Here's how the part is built. I have some questions about the finished solid (model axes, mm). Coordinates: 2 decimals unless noted, no trailing zeros. Order: outer loops, then holes, each group sorted by start corner. A loop starts at its lowest first (then second) coordinate and runs counter-clockwise, first axis right, second up. Notation, with made-up numbers: (83, -12.5) - (100, -12.5) arc R20 cw to (100, 19.5) - close; hole circle Ø10 at (18, 21). An arc over 180 degrees is marked (long way). Answer in a Markdown table with one row per item. Add a question column.
Item 1: I want a section at A-A (x = 31). Please give me the cut outline in (y, z).
Item 2: If I drill on line 1 along Y through (x, z) = (0, 0.7); line 2 along Y through (x, z) = (100, -0.65); line 3 along X through (y, z) = (-3.25, -1.2), over which ranges is the centre line in solid material (lowest first)? Write a range as from..to.
Item 3: I want a section at C-C (x = 93). Please give me the cut outline in (y, z), plus the area to 3 significant figures.
Item 4: Will this pin go through, and if not, where does the flat tip stop? pin 1 Ø1 at (y, z) = (9.5, -1) entering from -X.
Item 5: I want a section at D-D (y = -12.5). Please give me the cut outline in (x, z).
Item 6: I want a section at B-B (z = -0.85). Count the separate pieces of the cut face and the enclosed holes in it, plus the area to 3 significant figures.
```python
from build123d import *

# Parameters (mm, degrees)
BOSS_EXTRU_1_DEPTH      = 1.5
BOSS_EXTRU_1_DEPTH_BACK = 1.5
ESQUISSE1_R             = 0.8
ESQUISSE1_R_2           = 2.2
ESQUISSE1_R_3           = 4


with BuildPart() as part:
    # Esquisse1 → Boss.-Extru.1 (new, two sides: drawn at the far end of the back side and taken through both)
    with BuildSketch(Plane.XY.offset(-BOSS_EXTRU_1_DEPTH_BACK)):
        with BuildLine():
            Line((0, -15), (100, -10))
            ThreePointArc((100, -10), (110, 0), (100, 10))
            Line((100, 10), (0, 15))
            ThreePointArc((0, 15), (-15, 0), (0, -15))
        make_face()
        with Locations((5.656854249, 5.656854249)):
            Circle(ESQUISSE1_R, mode=Mode.SUBTRACT)
        with Locations((8, 0)):
            Circle(ESQUISSE1_R, mode=Mode.SUBTRACT)
        with Locations((5.656854249, -5.656854249)):
            Circle(ESQUISSE1_R, mode=Mode.SUBTRACT)
        with Locations((0, -8)):
            Circle(ESQUISSE1_R, mode=Mode.SUBTRACT)
        with Locations((100, 0)):
            Circle(ESQUISSE1_R_2, mode=Mode.SUBTRACT)
        Circle(ESQUISSE1_R_3, mode=Mode.SUBTRACT)
        with Locations((-5.656854249, -5.656854249)):
            Circle(ESQUISSE1_R, mode=Mode.SUBTRACT)
        with Locations((-8, 0)):
            Circle(ESQUISSE1_R, mode=Mode.SUBTRACT)
        with Locations((-5.656854249, 5.656854249)):
            Circle(ESQUISSE1_R, mode=Mode.SUBTRACT)
        with Locations((0, 8)):
            Circle(ESQUISSE1_R, mode=Mode.SUBTRACT)
        with BuildLine():
            Line((25.850093633, 7.7), (81.850093633, 4.9))
            ThreePointArc((81.850093633, 4.9), (86.750093633, 0), (81.850093633, -4.9))
            Line((81.850093633, -4.9), (25.850093633, -7.7))
            ThreePointArc((25.850093633, -7.7), (18.150093633, 0), (25.850093633, 7.7))
        make_face(mode=Mode.SUBTRACT)
    extrude(amount=BOSS_EXTRU_1_DEPTH + BOSS_EXTRU_1_DEPTH_BACK)


solid = part.part
```
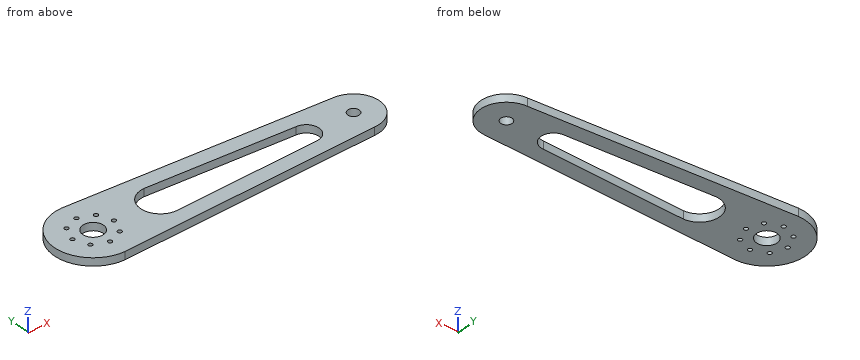
Values follow:
| question | item | result |
|---|---|---|
| 1 | outline | (-13.45, -1.5) - (-7.44, -1.5) - (-7.44, 1.5) - (-13.45, 1.5) - close; (7.44, -1.5) - (13.45, -1.5) - (13.45, 1.5) - (7.44, 1.5) - close |
| 2 | line 1 | y = -15..-8.8, -7.2..-4, 4..7.2, 8.8..15 |
| 2 | line 2 | y = -10..-2.2, 2.2..10 |
| 2 | line 3 | x = -14.64..-2.33, 2.33..18.87, 85.52..109.46 |
| 3 | outline | (-10.35, -1.5) - (10.35, -1.5) - (10.35, 1.5) - (-10.35, 1.5) - close |
| 3 | area | 62.1 mm^2 |
| 4 | pin 1 | stops at x = -12 |
| 5 | outline | (-8.29, -1.5) - (50, -1.5) - (50, 1.5) - (-8.29, 1.5) - close |
| 6 | separate pieces | 1 |
| 6 | enclosed holes | 11 |
| 6 | area | 2,090 mm^2 |
